Can you work these out from the drawing? Everything is in mm from the part's minimum corner. Give positions to 0.01 mm unless a question says otherwise; leave off trailing zeros. Use a Markdown table: item, result. Add a question column.
Item 1: I'm going to push flat-ended pins straight in: pin 1 Ø6 at (x, z) = (25.4, 76.2) entering from +Y; pin 2 Ø1 at (x, y) = (126, 4.5) entering from -Z (1 decimal); pin 3 Ø3 at (x, y) = (34.5, 2) entering from -Z. Where does each tip first touch, or does it pass through?
Item 2: If I drill on L1, parallel to X at y = 4, z = 76.2; L2, parallel to X at y = 1.5, z = 76.2; L3, parallel to X at y = 4.5, z = 89.5 (1 decimal), over which ranges is the centre line in solid material (lowest first)? Write a range as from..to.
Item 3: Suppose I cut it at A-A on z = 76.2. Count the separate pieces of the cut face and the enclosed holes in it, plus the area to 3 significant figures.
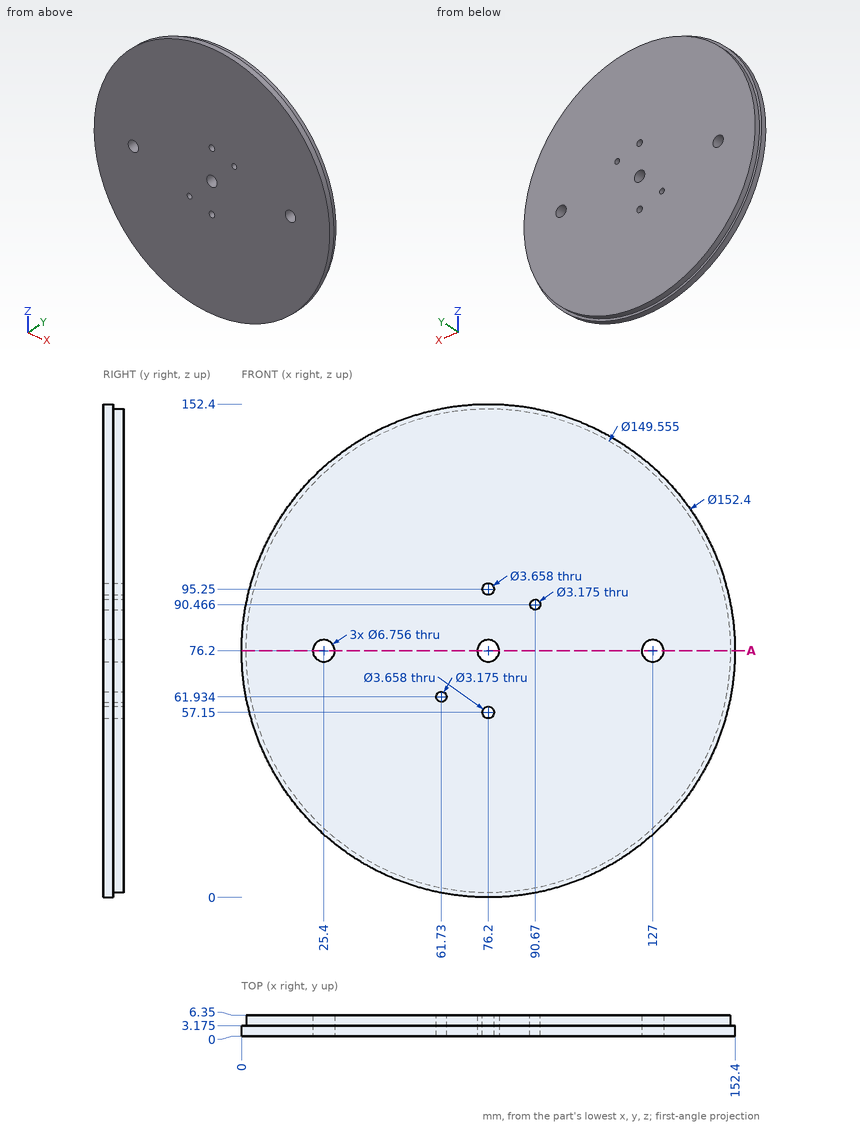
Findings below:
| question | item | result |
|---|---|---|
| 1 | pin 1 | passes through |
| 1 | pin 2 | stops at z = 20 |
| 1 | pin 3 | stops at z = 11.47 |
| 2 | L1 | x = 1.42..22.02, 28.78..72.82, 79.58..123.62, 130.38..150.98 |
| 2 | L2 | x = 0..22.02, 28.78..72.82, 79.58..123.62, 130.38..152.4 |
| 2 | L3 | x = 2.6..89.4, 91.9..149.8 |
| 3 | separate pieces | 4 |
| 3 | enclosed holes | 0 |
| 3 | area | 830 mm^2 |
